Geometry check sheet. Reference: the model listing, model coordinates, mm. A direction names the side the tool comes from. Give positions to 0.01 mm unless a question says otherwise; leave off trailing zeros. Write each loop counter-clockwise with the first axis right and the second up, starting at its lowest first coordinate (ties: lowest second). Pieces come first, ordered by that corner, then holes. Notation, with made-up numbers: (36, 77.5) - (43, 77.5) arc R19 ccw to (43, 106.5) - close; hole circle Ø9 at (7.25, -4). An arc over 180 degrees is marked (long way). One line per question, with ' | ' between items. Start each with the question number.
Q1. Section check A-A on x = 8. Record the boundary of the cut face in (y, z), and give its area (3 significant figures).
Q2. Section check C-C on x = -11. Record the boundary of the cut face in (y, z).
Q3. Section check D-D on y = -12.5. Record the boundary of the cut face in (x, z).
Q4. Thickness scan on L1, parallel to Z at x = -20, y = -10; L2, parallel to Z at x = -12, y = -5.5. Record the ranges inside material, lowest first. Write a range as [from, to].
Q5. Set-up check for faces 4 (the face through (-13, 0, 8.47)), 5 (the face through (2.6, 0.1, 8.97)): record each of +Z, -Z, +X, -X, +Y, -Y from which the full face is reachable in a straight line by a thin tool's end or side.
Q6. Section check B-B on y = 2. Record the boundary of the cut face in (x, z).
Q7. Release check for a two-part mould opening along Y. For faces 1 (the face through (8, 0, 8.67)), 2 (the face through (24, 0, 4)), 3 (the face through (0, -16.65, 4)) record: +Y half, -Y half, draft (parallel to the pull), parting line (faces both ways), or undercut.
Q8. Gauge pin test, flat ends, axial feed: P1, Ø3.5, axis at x = 9.5, y = -0.5, coming from the +Z side; P2, Ø3, axis at x = -13.5, y = 1, coming from the +Z side. Record the tip position at first contact, or that the pin passes through.
```python
from build123d import *

# Parameters (mm, degrees)
F0_W     = 48
F0_H     = 33.3
F1_DEPTH = 8.77
F2_W     = 7.6
F2_H     = 13.5
F2_W_2   = 5.58
F2_H_2   = 11.18
F3_DEPTH = 0.1
F4_DEPTH = 0.3
F5_W     = 13.07
F5_H     = 13.8
F5_W_2   = 11.15
F5_H_2   = 11.9
F6_DEPTH = 0.2
F7_DEPTH = 0.1


with BuildPart() as f1:
    # F0 (on Top) → F1 (new body)
    with BuildSketch(Plane.XY):
        Rectangle(F0_W, F0_H)
    extrude(amount=F1_DEPTH)

    # F2 (on face) → F3 (cut, symmetric)
    with BuildSketch(Plane.XY.offset(8.77)):
        with Locations((-12.83814013, 0)):
            Rectangle(F2_W, F2_H)
        with Locations((-12.83814013, 0)):
            Rectangle(F2_W_2, F2_H_2, mode=Mode.SUBTRACT)
    extrude(amount=F3_DEPTH, both=True, mode=Mode.SUBTRACT)

    # F4 (cut): a face of the model
    f4_faces = [f1.faces().sort_by_distance(p)[0] for p in [
        (-12.83814013, 0, 8.77),
    ]]
    extrude(f4_faces, amount=-F4_DEPTH, mode=Mode.SUBTRACT)

    # F5 (on face) → F6 (join)
    with BuildSketch(Plane.XY.offset(8.77)):
        with Locations((8.4796537594, 0)):
            Rectangle(F5_W, F5_H)
        with Locations((8.4796537594, 0)):
            Rectangle(F5_W_2, F5_H_2, mode=Mode.SUBTRACT)
    extrude(amount=F6_DEPTH)

    # F7 (cut): a face of the model
    f7_faces = [f1.faces().sort_by_distance(p)[0] for p in [
        (8.4796537594, 0, 8.77),
    ]]
    extrude(f7_faces, amount=-F7_DEPTH, mode=Mode.SUBTRACT)


solid = f1.part
```
Working result:
1) outline: (-16.65, 0) - (16.65, 0) - (16.65, 8.77) - (6.9, 8.77) - (6.9, 8.97) - (5.95, 8.97) - (5.95, 8.67) - (-5.95, 8.67) - (-5.95, 8.97) - (-6.9, 8.97) - (-6.9, 8.77) - (-16.65, 8.77) - close | area: 291 mm2
2) outline: (-16.65, 0) - (16.65, 0) - (16.65, 8.77) - (6.75, 8.77) - (6.75, 8.67) - (5.59, 8.67) - (5.59, 8.47) - (-5.59, 8.47) - (-5.59, 8.67) - (-6.75, 8.67) - (-6.75, 8.77) - (-16.65, 8.77) - close
3) outline: (-24, 0) - (24, 0) - (24, 8.77) - (-24, 8.77) - close
4) L1: z = [0, 8.77] | L2: z = [0, 8.47]
5) face 4: +Z | face 5: +Z, +X, -X, +Y, -Y
6) outline: (-24, 0) - (24, 0) - (24, 8.77) - (15.01, 8.77) - (15.01, 8.97) - (14.05, 8.97) - (14.05, 8.67) - (2.9, 8.67) - (2.9, 8.97) - (1.94, 8.97) - (1.94, 8.77) - (-9.04, 8.77) - (-9.04, 8.67) - (-10.05, 8.67) - (-10.05, 8.47) - (-15.63, 8.47) - (-15.63, 8.67) - (-16.64, 8.67) - (-16.64, 8.77) - (-24, 8.77) - close
7) face 1: undercut | face 2: draft | face 3: -Y half
8) P1: stops at z = 8.67 | P2: stops at z = 8.47
